CAD build for the part. Positions are in the model's coordinates, mm. A direction names the side the tool comes from. Give positions to 0.01 mm unless a question says otherwise; leave off trailing zeros. Order: outer loops, then holes, each group sorted by start corner. A loop starts at its lowest first (then second) coordinate and runs counter-clockwise, first axis right, second up.
```python
from build123d import *

# Parameters (mm, degrees)
F1_DEPTH  = 10.2
F2_W      = 28.5
F2_H      = 27.5
F2_W_2    = 19.5
F2_H_2    = 19.5
F3_DEPTH  = 2
F4_R      = 1.9685
F5_DEPTH  = 38.5
F6_W      = 5
F6_H      = 6
F7_DEPTH  = 2
F8_W      = 5
F8_H      = 6
F9_DEPTH  = 2
F10_W     = 1
F10_H     = 8.25
F11_DEPTH = 0.5
F12_R     = 2.5
F13_DEPTH = 12.201


with BuildPart() as f1:
    # F0 (on Front) → F1 (new body)
    with BuildSketch(Plane.XZ):
        with BuildLine():
            Line((-14.25, 3), (-19.25, 3))
            Line((-19.25, 3), (-19.25, 0))
            Line((-19.25, 0), (-13.75, 0))
            ThreePointArc((-13.75, 0), (-13.017766953, 1.767766953), (-11.25, 2.5))
            Line((-11.25, 2.5), (-11.25, 10.75))
            Line((-11.25, 10.75), (0, 10.75))
            Line((0, 10.75), (0, 13.75))
            Line((0, 13.75), (-14.25, 13.75))
            Line((-14.25, 13.75), (-14.25, 3))
        make_face()
        with BuildLine():
            Line((-13.75, 0), (-19.25, 0))
            Line((-19.25, 0), (-19.25, -3))
            Line((-19.25, -3), (-14.25, -3))
            Line((-14.25, -3), (-14.25, -13.75))
            Line((-14.25, -13.75), (0, -13.75))
            Line((0, -13.75), (0, -10.75))
            Line((0, -10.75), (-11.25, -10.75))
            Line((-11.25, -10.75), (-11.25, -2.5))
            ThreePointArc((-11.25, -2.5), (-13.017766953, -1.767766953), (-13.75, 0))
        make_face()
        with BuildLine():
            Line((14.25, 13.75), (0, 13.75))
            Line((0, 13.75), (0, 10.75))
            Line((0, 10.75), (11.25, 10.75))
            Line((11.25, 10.75), (11.25, 2.5))
            ThreePointArc((11.25, 2.5), (13.017766953, 1.767766953), (13.75, 0))
            Line((13.75, 0), (19.25, 0))
            Line((19.25, 0), (19.25, 3))
            Line((19.25, 3), (14.25, 3))
            Line((14.25, 3), (14.25, 13.75))
        make_face()
        with BuildLine():
            Line((11.25, -10.75), (0, -10.75))
            Line((0, -10.75), (0, -13.75))
            Line((0, -13.75), (14.25, -13.75))
            Line((14.25, -13.75), (14.25, -3))
            Line((14.25, -3), (19.25, -3))
            Line((19.25, -3), (19.25, 0))
            Line((19.25, 0), (13.75, 0))
            ThreePointArc((13.75, 0), (13.017766953, -1.767766953), (11.25, -2.5))
            Line((11.25, -2.5), (11.25, -10.75))
        make_face()
    extrude(amount=F1_DEPTH)

    # F2 (on face) → F3 (join)
    with BuildSketch(Plane(origin=(0, 0, 0), x_dir=(-1, 0, 0), z_dir=(0, 1, 0))):
        Rectangle(F2_W, F2_H)
        Rectangle(F2_W_2, F2_H_2, mode=Mode.SUBTRACT)
    extrude(amount=F3_DEPTH)

    # F4 (on face) → F5 (cut, through all)
    with BuildSketch(Plane(origin=(-19.25, 0, 0), x_dir=(0, -1, 0), z_dir=(-1, 0, 0))):
        with Locations((5.1, 0)):
            Circle(F4_R)
    extrude(amount=-F5_DEPTH, mode=Mode.SUBTRACT)

    # F6 (on face) → F7 (join, through all)
    with BuildSketch(Plane(origin=(0, 0, 0), x_dir=(-1, 0, 0), z_dir=(0, 1, 0))):
        with Locations((-16.75, 0)):
            Rectangle(F6_W, F6_H)
    extrude(amount=F7_DEPTH)

    # F8 (on face) → F9 (join, through all)
    with BuildSketch(Plane(origin=(0, 0, 0), x_dir=(-1, 0, 0), z_dir=(0, 1, 0))):
        with Locations((16.75, 0)):
            Rectangle(F8_W, F8_H)
    extrude(amount=F9_DEPTH)

    # F10 (on face) → F11 (join)
    with BuildSketch(Plane.XZ.offset(10.2)):
        with Locations((-10.75, 6.625)):
            Rectangle(F10_W, F10_H)
        with Locations((10.75, 6.625)):
            Rectangle(F10_W, F10_H)
        with Locations((-10.75, -6.625)):
            Rectangle(F10_W, F10_H)
        with Locations((10.75, -6.625)):
            Rectangle(F10_W, F10_H)
    extrude(amount=-F11_DEPTH)

    # F12 (on face) → F13 (cut, through all)
    with BuildSketch(Plane.XZ.offset(10.2)):
        with Locations((-11.25, 0)):
            Circle(F12_R)
        with Locations((11.25, 0)):
            Circle(F12_R)
    extrude(amount=-F13_DEPTH, mode=Mode.SUBTRACT)


solid = f1.part
```
Item 1: Two-plate mould, pull along Y, no slides. Class faces 1 (the face through (0, 1, 9.75)), 2 (the face through (0, -10.2, -12)), 3 (the face through (0, 0, 10)): released by +Y, released by -Y, zero draft, split by the parting line, or undercut.
Item 2: Slice it at A-A (y = -5.1). Give the cut face in (x, z).
Item 3: Tool access for faces 4 (the face through (-9.75, 1, 6)), 5 (the face through (-11, -9.7, -7)), 6 (the face through (17, -4, -3)), 7 (the face through (-14.25, -4, 8)): list every direction of +Z, -Z, +X, -X, +Y, -Y with a clear straight run to the whole face (end or side of a thin tool).
Item 4: Slice it at D-D (y = -2.5). Give the cut face in (x, z), and give its area (3 significant figures).
Item 5: Wall check: L1, parallel to X at y = -9.5, z = -4; L2, parallel to X at y = 0.85, z = 0; L3, parallel to Z at x = -11.25, y = 1.45. Give the ranges that are in metal, low to high.
Item 6: Slice it at B-B (x = -4). Give the cut face in (y, z), and give its area (3 significant figures).
Item 7: Slice it at C-C (z = -6.25). Give the cut face in (x, y), and give its area (3 significant figures).
Item 8: Drop flat-ended pins along their axis: pin 1 Ø10 at (x, z) = (-9.5, 0.5) entering from +Y; pin 2 Ø2 at (y, z) = (-7.5, -6.5) entering from -X; pin 3 Ø2.5 at (y, z) = (-3.5, 5) entering from +X; pin 4 Ø2.5 at (x, y) = (-16, -5.5) entering from -Z. Give the stop position or say it passes through.
A:
1. face 1: zero draft
1. face 2: released by -Y
1. face 3: undercut
2. outline: (-19.25, -3) - (-14.25, -3) - (-14.25, -13.75) - (14.25, -13.75) - (14.25, -3) - (19.25, -3) - (19.25, -1.97) - (12.79, -1.97) arc R2.5 cw to (11.25, -2.5) - (11.25, -10.75) - (-11.25, -10.75) - (-11.25, -2.5) arc R2.5 cw to (-12.79, -1.97) - (-19.25, -1.97) - close; (-19.25, 1.97) - (-12.79, 1.97) arc R2.5 cw to (-11.25, 2.5) - (-11.25, 10.75) - (11.25, 10.75) - (11.25, 2.5) arc R2.5 cw to (12.79, 1.97) - (19.25, 1.97) - (19.25, 3) - (14.25, 3) - (14.25, 13.75) - (-14.25, 13.75) - (-14.25, 3) - (-19.25, 3) - close
3. face 4: +Y, -Y
3. face 5: none
3. face 6: -Z, +X, +Y, -Y
3. face 7: +Z, -X, +Y, -Y
4. outline: (-19.25, -3) - (-14.25, -3) - (-14.25, -13.75) - (14.25, -13.75) - (14.25, -3) - (19.25, -3) - (19.25, 3) - (14.25, 3) - (14.25, 13.75) - (-14.25, 13.75) - (-14.25, 3) - (-19.25, 3) - close; hole (-11.25, -10.75) - (11.25, -10.75) - (11.25, -2.5) arc R2.5 ccw to (11.25, 2.5) - (11.25, 10.75) - (-11.25, 10.75) - (-11.25, 2.5) arc R2.5 ccw to (-11.25, -2.5) - close
4. area: 340 mm2
5. L1: x = -14.25 to -11.25, 11.25 to 14.25
5. L2: x = -19.25 to -13.75, 13.75 to 19.25
5. L3: z = -13.75 to -2.5, 2.5 to 13.75
6. outline: (-10.2, -13.75) - (2, -13.75) - (2, -9.75) - (0, -9.75) - (0, -10.75) - (-10.2, -10.75) - close; (-10.2, 10.75) - (0, 10.75) - (0, 9.75) - (2, 9.75) - (2, 13.75) - (-10.2, 13.75) - close
6. area: 77.2 mm2
7. outline: (-14.25, -10.2) - (-10.25, -10.2) - (-10.25, -9.7) - (-11.25, -9.7) - (-11.25, 0) - (-9.75, 0) - (-9.75, 2) - (-14.25, 2) - close; (9.75, 0) - (11.25, 0) - (11.25, -9.7) - (10.25, -9.7) - (10.25, -10.2) - (14.25, -10.2) - (14.25, 2) - (9.75, 2) - close
7. area: 80.2 mm2
8. pin 1: stops at y = 2
8. pin 2: stops at x = -14.25
8. pin 3: stops at x = 14.25
8. pin 4: stops at z = -3
